Check sheet for the modelled part. Datum: model origin and axes. Units: mm. A direction names the side the tool comes from. Round coordinates to 2 decimals unless told otherwise and drop trailing zeros. Loops run counter-clockwise (first coordinate to the right, second up) from the corner with the lowest first, then second, coordinate; pieces in that order, holes last. Notation, with made-up numbers: (-19.5, -23) - (-2.5, -23) arc R21 ccw to (-2.5, -18) - close; hole circle Ø11 at (81, -29). An arc over 180 degrees is marked (long way). Answer in a Markdown table with one row per item. Add a question column.
(1) Cross-section at B-B on x = -6. Enter the section's corners in (y, z).
(2) Thickness scan on line 1 along X through (y, z) = (-35.5, 114); line 2 along Y through (x, z) = (-118, 98.5); line 3 along Z through (x, y) = (-1.5, -19). Record the ranges inside material, lowest first.
(3) Cross-section at D-D on x = -80. Enter the section's corners in (y, z), then the cut area to 3 significant figures.
(4) Access from +Z, -Z, +X, -X, +Y, -Y to the whole of each face (thin tool, end or side, straight path). Record for faces 3 (the flat face through (-68, -66.66, 3)), 4 (the flat face through (-20, -74.66, 77)).
(5) Cross-section at C-C on y = -23. Count the separate pieces of the cut face and the enclosed holes in it, then the cut area to 3 significant figures.
(6) Cross-section at A-A on z = 91. Enter the section's corners in (x, y).
(7) Mould release check, pull along X, two halves, no side actions. Record for faces 1 (the flat face through (-20, -1, 0)), 2 (the flat face through (-93.322, -3, 3)): +X half, -X half, draft (parallel to the pull), parting line (faces both ways), or undercut.
from build123d import *

# Parameters (mm, degrees)
F1_W     = 246
F1_H     = 146
F1_W_2   = 10
F1_H_2   = 130
F2_DEPTH = 6
F3_DEPTH = 150


# Not quite as in the source:
# - ends of sketch curves that miss each other by under 0.0002 mm in the source are joined


with BuildPart() as f2:
    # F1 (on face) → F2 (new body)
    with BuildSketch(Plane.XY):
        with Locations((-18.3215842792, -1.6598337144)):
            Rectangle(F1_W, F1_H)
        with Locations((-128.3215842792, -1.6598337144)):
            Rectangle(F1_W_2, F1_H_2, mode=Mode.SUBTRACT)
        with Locations((-108.3215842792, -1.6598337144)):
            Rectangle(F1_W_2, F1_H_2, mode=Mode.SUBTRACT)
        with Locations((-88.3215842792, -1.6598337144)):
            Rectangle(F1_W_2, F1_H_2, mode=Mode.SUBTRACT)
        with Locations((-68.3215842792, -1.6598337144)):
            Rectangle(F1_W_2, F1_H_2, mode=Mode.SUBTRACT)
        with Locations((-48.3215842792, -1.6598337144)):
            Rectangle(F1_W_2, F1_H_2, mode=Mode.SUBTRACT)
        with Locations((-28.3215842792, -1.6598337144)):
            Rectangle(F1_W_2, F1_H_2, mode=Mode.SUBTRACT)
        with Locations((-8.3215842792, -1.6598337144)):
            Rectangle(F1_W_2, F1_H_2, mode=Mode.SUBTRACT)
        with Locations((11.6784157208, -1.6598337144)):
            Rectangle(F1_W_2, F1_H_2, mode=Mode.SUBTRACT)
        with Locations((31.6784157208, -1.6598337144)):
            Rectangle(F1_W_2, F1_H_2, mode=Mode.SUBTRACT)
        with Locations((51.6784157208, -1.6598337144)):
            Rectangle(F1_W_2, F1_H_2, mode=Mode.SUBTRACT)
        with Locations((71.6784157208, -1.6598337144)):
            Rectangle(F1_W_2, F1_H_2, mode=Mode.SUBTRACT)
        with Locations((91.6784157208, -1.6598337144)):
            Rectangle(F1_W_2, F1_H_2, mode=Mode.SUBTRACT)
    extrude(amount=F2_DEPTH)

    # F1 (on face) → F3 (join)
    with BuildSketch(Plane.XY):
        Polygon((106.6783964634, -76.6597911716), (106.6783964634, 73.3401662856), (-143.3215842792, 73.3401662856), (-143.3215842792, -76.6598337144), align=None)
        with Locations((-18.3215842792, -1.6598337144)):
            Rectangle(F1_W, F1_H, mode=Mode.SUBTRACT)
    extrude(amount=F3_DEPTH)


solid = f2.part
Answers:
| question | item | result |
|---|---|---|
| 1 | outline | (-76.66, 0) - (-66.66, 0) - (-66.66, 6) - (-74.66, 6) - (-74.66, 150) - (-76.66, 150) - close; (63.34, 0) - (73.34, 0) - (73.34, 150) - (71.34, 150) - (71.34, 6) - (63.34, 6) - close |
| 2 | line 1 | x = -143.32 to -141.32, 104.68 to 106.68 |
| 2 | line 2 | y = -76.66 to -74.66, 71.34 to 73.34 |
| 2 | line 3 | z = 0 to 6 |
| 3 | outline | (-76.66, 0) - (73.34, 0) - (73.34, 150) - (71.34, 150) - (71.34, 6) - (-74.66, 6) - (-74.66, 150) - (-76.66, 150) - close |
| 3 | area | 1,480 mm^2 |
| 4 | face 3 | +Z, -Z |
| 4 | face 4 | +Z |
| 5 | separate pieces | 13 |
| 5 | enclosed holes | 0 |
| 5 | area | 1,360 mm^2 |
| 6 | outline | (-143.32, -76.66) - (106.68, -76.66) - (106.68, 73.34) - (-143.32, 73.34) - close; hole (-141.32, -74.66) - (104.68, -74.66) - (104.68, 71.34) - (-141.32, 71.34) - close |
| 7 | face 1 | draft |
| 7 | face 2 | undercut |
